Design review of the part shown in the three views and the two pictorial views. Dimensions are in mm from the part's minimum x, y and z. Give positions to 0.01 mm unless a question says otherwise; leave off trailing zeros. Order: outer loops, then holes, each group sorted by start corner. A loop starts at its lowest first (then second) coordinate and runs counter-clockwise, first axis right, second up. Notation, with made-up numbers: M 69,-5.5 L 110,-5.5 A12 cw 110,4.5 Z; hole C 9,17.5 d7. An arc over 180 degrees is marked long. Answer as a JSON object with one key per item and string values.
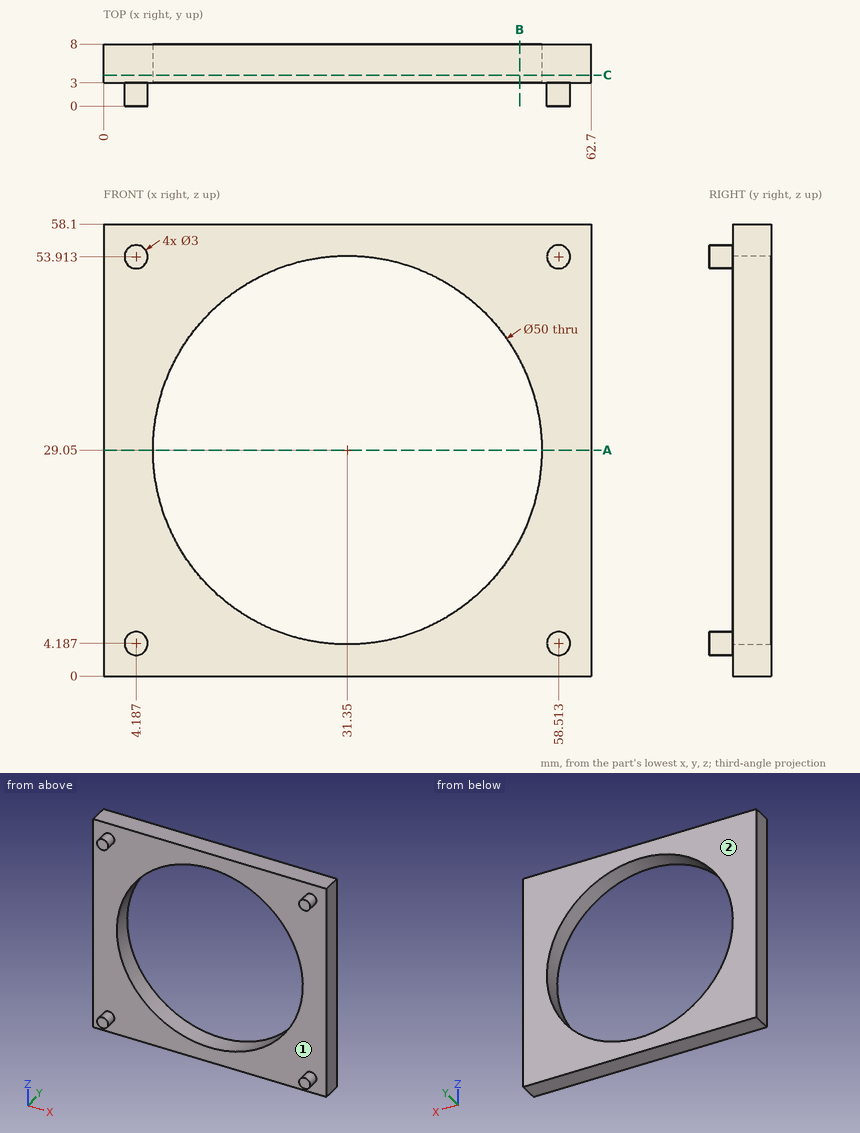
(1) We need section B-B (x = 53.5). Write out the cut boundary in (y, z), plus the area to 3 significant figures.
Checked values:
{"outline": "M 3,0 L 8,0 L 8,17.46 L 3,17.46 Z; M 3,40.64 L 8,40.64 L 8,58.1 L 3,58.1 Z", "area": "175 mm^2"}
(2) We need section C-C (y = 4). Write out the cut boundary in (x, z).
Checked values:
{"outline": "M 0,0 L 62.7,0 L 62.7,58.1 L 0,58.1 Z; hole C 31.35,29.05 d50"}
(3) We need section A-A (z = 29.05). Write out the cut boundary in (x, y), plus the area to 3 significant figures.
Checked values:
{"outline": "M 0,3 L 6.35,3 L 6.35,8 L 0,8 Z; M 56.35,3 L 62.7,3 L 62.7,8 L 56.35,8 Z", "area": "63.5 mm^2"}
(4) To check wall thickness, follow L1, parallel to X at y = 5.2, z = 29.05; L2, parallel to X at y = 2.5, z = 4 (1 decimal); L3, parallel to Z at x = 44.5, y = 5.25. State the ranges of each line that lie inside material, in increasing order. Write a range as from..to.
Checked values:
{"L1": "x = 0..6.35, 56.35..62.7", "L2": "x = 2.7..5.7, 57..60", "L3": "z = 0..7.79, 50.31..58.1"}
(5) Draft analysis for pull direction Z (two halves, no side actions). For the marked faces 1 and 2, state which applies: +Z half, -Z half, draft (parallel to the pull), parting line (faces both ways), or undercut.
Checked values:
{"face 1": "undercut", "face 2": "draft"}
